```python
from build123d import *

# Parameters (mm, degrees)
BOSS_EXTRUDE1_DEPTH     = 12.7
SKETCH3_W               = 47.23204247
SKETCH3_H               = 13.081
CUT_EXTRUDE1_DEPTH      = 924.408729549
BOSS_EXTRUDE3_DEPTH     = 12.7
F_1_4_CLEARANCE_HOLE1_D = 6.7564
SKETCH13_W              = 23.41954247
SKETCH13_H              = 28.3464
CUT_EXTRUDE2_DEPTH      = 924.408729549
SKETCH14_R              = 3.429
CUT_EXTRUDE3_DEPTH      = 913.678476707
FILLET4_R               = 50.8
FILLET5_R               = 12.7
FILLET6_R               = 1.27
FILLET7_R               = 0.508
F_1_4_CLEARANCE_HOLE2_D = 6.7564
CUT_EXTRUDE4_DEPTH      = 913.678476707
FILLET8_R               = 1.27


with BuildPart() as part:
    # Sketch1 → Boss-Extrude1 (new body)
    with BuildSketch(Plane.XY):
        Polygon((0, 0), (-396.875, 787.4), (-482.20704247, 787.4), (-85.33204247, 0), align=None)
    extrude(amount=BOSS_EXTRUDE1_DEPTH)

    # Sketch3 → Cut-Extrude1 (cut, through all)
    with BuildSketch(Plane.XY.offset(12.7)):
        with Locations((-252.216021235, 371.4115)):
            Rectangle(SKETCH3_W, SKETCH3_H)
        with Locations((-444.303521235, 752.5131)):
            Rectangle(SKETCH3_W, SKETCH3_H)
    extrude(amount=-CUT_EXTRUDE1_DEPTH, mode=Mode.SUBTRACT)

    # Sketch10 → Boss-Extrude3 (add)
    with BuildSketch(Plane.XY.offset(12.7)):
        with BuildLine():
            Line((-244.024703128, 501.780299783), (-249.740869802, 513.121174464))
            ThreePointArc((-249.740869802, 513.121174464), (-246.928515798, 521.649695143), (-238.39999512, 518.837341139))
            Line((-238.39999512, 518.837341139), (-226.967661771, 496.155591775))
            Line((-226.967661771, 496.155591775), (-239.680416455, 475.525946247))
            Line((-239.680416455, 475.525946247), (-251.112749804, 498.207695611))
            ThreePointArc((-251.112749804, 498.207695611), (-245.78242438, 496.449974359), (-244.024703128, 501.780299783))
        make_face()
        with BuildLine():
            Line((-351.145666605, 696.673002545), (-362.577999954, 719.354751908))
            ThreePointArc((-362.577999954, 719.354751908), (-357.24767453, 717.597030656), (-355.489953278, 722.92735608))
            Line((-355.489953278, 722.92735608), (-361.206119952, 734.268230762))
            ThreePointArc((-361.206119952, 734.268230762), (-358.393765948, 742.79675144), (-349.86524527, 739.984397436))
            Line((-349.86524527, 739.984397436), (-338.432911921, 717.302648072))
            Line((-338.432911921, 717.302648072), (-351.145666605, 696.673002545))
        make_face()
        with BuildLine():
            Line((0, 0), (-11.432333349, 22.681749364))
            ThreePointArc((-11.432333349, 22.681749364), (-6.102007925, 20.924028111), (-4.344286673, 26.254353535))
            Line((-4.344286673, 26.254353535), (-10.060453347, 37.595228217))
            ThreePointArc((-10.060453347, 37.595228217), (-7.248099343, 46.123748895), (1.280421335, 43.311394892))
            Line((1.280421335, 43.311394892), (12.712754684, 20.629645528))
            Line((12.712754684, 20.629645528), (23.110761502, 0))
            Line((23.110761502, 0), (0, 0))
        make_face()
    extrude(amount=-BOSS_EXTRUDE3_DEPTH)

    # 1/4 Clearance Hole1 (through all)
    with Locations(Plane.XY.offset(12.7)):
        with Locations((-99.918593468, 162.967911886), (-427.0375, 720.5726), (-395.2875, 720.5726), (-203.2, 339.471), (-234.95, 339.471), (-69.85, 25.4), (-38.1, 25.4)):
            Hole(F_1_4_CLEARANCE_HOLE1_D / 2)

    # Sketch13 → Cut-Extrude2 (cut, through all)
    with BuildSketch(Plane.XY.offset(12.7)):
        with Locations((-470.497271235, 773.2268)):
            Rectangle(SKETCH13_W, SKETCH13_H)
    extrude(amount=-CUT_EXTRUDE2_DEPTH, mode=Mode.SUBTRACT)

    # Sketch14 → Cut-Extrude3 (cut, through all)
    with BuildSketch(Plane.XY.offset(12.7)):
        with Locations((-424.1165, 759.0536)):
            Circle(SKETCH14_R)
        with Locations((-424.1165, 745.9726)):
            Circle(SKETCH14_R)
        with Locations((-232.029, 377.952)):
            Circle(SKETCH14_R)
        with Locations((-232.029, 364.871)):
            Circle(SKETCH14_R)
    extrude(amount=-CUT_EXTRUDE3_DEPTH, mode=Mode.SUBTRACT)

    # Fillet4
    # the kernel refuses this fillet: 50.8 mm, written as the material it adds along each edge
    with BuildSketch(Plane(origin=(-239.680416455, 475.525946247, 12.7), x_dir=(0.45009186412240076, -0.8929822584188458, 0), z_dir=(0, 0, -1))) as fillet4_piece_1:
        with BuildLine():
            CenterArc((28.176198377, -50.8), FILLET4_R, 90, 53.576426358)
            Line((-12.7, -20.6375), (-13.517523968, -20.03425))
            ThreePointArc((-13.517523968, -20.03425), (-7.21528485, -9.786267016), (-0.86528485, 0.532482984))
            Line((-0.86528485, 0.532482984), (0, 1.016))
            Line((0, 1.016), (28.176198377, 1.016))
            Line((28.176198377, 1.016), (28.176198377, 0))
        make_face()
    extrude(amount=12.7)

    # Fillet5
    fillet5_edges = [part.edges().sort_by_distance(p)[0] for p in [
        (-458.7875, 787.4, 6.35),
        (-226.967661771, 496.155591775, 6.35),
        (-338.432911921, 717.302648072, 6.35),
        (-351.145666605, 696.673002545, 6.35),
    ]]
    fillet(fillet5_edges, radius=FILLET5_R)

    # Fillet6
    fillet6_edges = [part.edges().sort_by_distance(p)[0] for p in [
        (-458.7875, 759.0536, 6.35),
        (-269.238796502, 364.871, 6.35),
        (-275.83204247, 377.952, 6.35),
    ]]
    fillet(fillet6_edges, radius=FILLET6_R)

    # Fillet7
    fillet7_edges = [part.edges().sort_by_distance(p)[0] for p in [
        (-235.458, 377.952, 6.35),
        (-427.5455, 759.0536, 6.35),
        (-427.5455, 745.9726, 6.35),
        (-235.458, 364.871, 6.35),
    ]]
    fillet(fillet7_edges, radius=FILLET7_R)

    # 1/4 Clearance Hole2 (through all)
    with Locations(Plane.XY.offset(12.7)):
        with Locations((-447.675, 736.6), (-449.2625, 774.7)):
            Hole(F_1_4_CLEARANCE_HOLE2_D / 2)

    # Sketch18 → Cut-Extrude4 (cut, through all)
    with BuildSketch(Plane.XY.offset(12.7)):
        Polygon((-458.7875, 745.9726), (-458.7875, 740.93562774), (-461.326296502, 745.9726), align=None)
    extrude(amount=-CUT_EXTRUDE4_DEPTH, mode=Mode.SUBTRACT)

    # Fillet8
    fillet8_edges = [part.edges().sort_by_distance(p)[0] for p in [
        (-458.7875, 745.9726, 6.35),
        (-458.7875, 740.93562774, 6.35),
        (-85.33204247, 0, 6.35),
        (23.110761502, 0, 6.35),
        (-396.875, 787.4, 6.35),
    ]]
    fillet(fillet8_edges, radius=FILLET8_R)


solid = part.part
```
Input: part model. Units: mm. Frame: model coordinates. Round coordinates to 2 decimals unless told otherwise and drop trailing zeros. Order: outer loops, then holes, each group sorted by start corner. A loop starts at its lowest first (then second) coordinate and runs counter-clockwise, first axis right, second up. Notation, with made-up numbers: (-23, -5) - (-7, -5) arc R21 ccw to (-7, 28) - close; hole circle Ø9 at (0.5, -16.5). An arc over 180 degrees is marked (long way). One line per question, with ' | ' between items. Start each with the question number.
1) Contact query for flat-ended pins moving along their axis: P1, Ø4, axis at x = -216, z = 3.5, coming from the +Y side; P2, Ø5, axis at y = 566, z = 9, coming from the +X side; P3, Ø6, axis at x = -449.26, y = 774.7, coming from the -Z side; P4, Ø4, axis at x = -449.5, z = 8.5, coming from the +Y side. Output: stop coordinate, or through.
2) Pull-direction query (X, two-part tool) for faces 1 (the flat face through (-379.313, 752.557, 6.261)), 2 (the flat face through (-178.276, 184.4, 6.261)), 3 (the flat face through (-224, 381, 12.7)); classes: +X half, -X half, draft (parallel to the pull), parting line (faces both ways), or undercut.
3) Cut plane A-A, the plane x = -376. Return the cut outline in (y, z).
4) Cut plane B-B, the plane z = 9.5. Give the number of separate pieces and of enclosed holes in the cut face, then the cut area to 3 significant figures.
5) Ray query, probe 1 along X at (y, z) = (340, 1.5); probe 2 along X at (y, z) = (736.6, 8); probe 3 along X at (y, z) = (724, 8). Return the intervals inside material, ascending.
6) Cut plane C-C, the plane y = 651.5. Return the cut outline in (x, z), then the cut area to 3 significant figures.
Worked out:
1) P1: stops at y = 432.51 | P2: stops at x = -284.02 | P3: passes through | P4: stops at y = 787.32
2) face 1: undercut | face 2: -X half | face 3: draft
3) outline: (576.69, 0) - (745.98, 0) - (745.98, 12.7) - (576.69, 12.7) - close
4) separate pieces: 1 | enclosed holes: 9 | area: 67,300 mm^2
5) probe 1: x = -256.7 to -238.29, -231.61 to -206.54, -199.86 to -171.37 | probe 2: x = -456.6 to -451.05, -444.3 to -371.27, -361.86 to -348.16 | probe 3: x = -450.25 to -364.92, -356.03 to -341.81
6) outline: (-413.71, 0) - (-328.38, 0) - (-328.38, 12.7) - (-413.71, 12.7) - close | area: 1,080 mm^2
